from build123d import *

# Parameters (mm, degrees)
CYLINDER072_R               = 42
CYLINDER072_DEPTH           = 297
CYLINDER073_W               = 46
CYLINDER073_H               = 280
CYLINDER073_ANGLE           = 230
CYLINDER073_PLACEMENT_ANGLE = 184


with BuildPart() as cylindre068:
    # Cylinder072 → Cylinder072 (new body)
    with BuildSketch(Plane.XY.offset(-207)):
        Circle(CYLINDER072_R)
    extrude(amount=CYLINDER072_DEPTH)


with BuildPart() as obj1:
    # Cylinder073 → Cylinder073 (revolve)
    with BuildSketch(Plane.XZ):
        with Locations((23, 140)):
            Rectangle(CYLINDER073_W, CYLINDER073_H)
    revolve(axis=Axis((0, 0, 0), (0, 0, 1)), revolution_arc=CYLINDER073_ANGLE)


with BuildPart() as obj1_1:
    # Cylinder073 placement: moved
    add(obj1.part.moved(Location((0, 0, -207))).rotate(Axis((0, 0, -207), (0, 0, 1)), CYLINDER073_PLACEMENT_ANGLE))

    # Cut041: cut Cylindre068
    add(cylindre068.part, mode=Mode.SUBTRACT)


with BuildPart() as obj1_2:
    # Cut041 placement: moved
    add(obj1_1.part.moved(Location((0, 0, 8))))


solid = obj1_2.part
Can you work these out from the model? Positions are in its coordinate system, mm. Coordinates: 2 decimals unless noted, no trailing zeros. Loops run counter-clockwise (first coordinate to the right, second up) from the corner with the lowest first, then second, coordinate; pieces in that order, holes last. Notation, with made-up numbers: (62.25, -40) - (94.25, -40) arc R25 ccw to (94.25, -16) - close; hole circle Ø9 at (38.5, 15). An arc over 180 degrees is marked (long way). Put each result on its own line as item: value. Start each with the question number.
Item 1: If I drill on line 1 along Y through (x, z) = (0, -15.5); line 2 along X through (y, z) = (1, -125); line 3 along X through (y, z) = (-38.5, -93), over which ranges is the centre line in solid material (lowest first)?
Item 2: Suppose I cut it at A-A (y = -11.5). Please give me the cut outline in (x, z), and give its area (3 significant figures).
Item 3: If we mould it in two halves opening along X, with no side actions, what happens to faces 1 (the face through (19.5, -37.4, 81)), 2 (the face through (21.162, -40.843, -57.04)), 3 (the face through (19.322, -37.292, -60.96))? For each: +X half, -X half, draft (parallel to the pull), parting line (faces both ways), or undercut.
Item 4: For pin 1 (3 mm diameter, centred on y = -11.5, z = -24, fed in from -X); pin 2 (6 mm diameter, centred on y = 23, z = -4.5, fed in from +X); pin 3 (12 mm diameter, centred on x = -16, z = -158.5, fed in from -Y), each with a flat end and sliding along its axis, tell me the tip position at first contact or that it passes through.
Item 5: Suppose I cut it at C-C (x = 0). Please give me the cut outline in (y, z), and give its area (3 significant figures).
Item 6: Suppose I cut it at D-D (z = -137). Please give me the cut outline in (x, y).
Item 7: Suppose I cut it at B-B (x = 39.5). Please give me the cut outline in (y, z), and give its area (3 significant figures).
Here are the results:
1. line 1: -46 to -42
1. line 2: 41.99 to 45.99
1. line 3: -25.17 to -16.79, 16.79 to 25.17
2. outline: (-44.54, -199) - (-40.39, -199) - (-40.39, 81) - (-44.54, 81) - close; (40.39, -199) - (44.54, -199) - (44.54, 81) - (40.39, 81) - close
2. area: 2,320 mm²
3. face 1: draft
3. face 2: parting line
3. face 3: undercut
4. pin 1: x = -44.9
4. pin 2: x = 41.42
4. pin 3: y = -44.9
5. outline: (-46, -199) - (-42, -199) - (-42, 81) - (-46, 81) - close
5. area: 1,120 mm²
6. outline: (-45.89, -3.21) arc R46 ccw (long way) to (27.04, 37.21) - (24.69, 33.98) arc R42 cw (long way) to (-41.9, -2.93) - close
7. outline: (-23.57, -199) - (-14.27, -199) - (-14.27, 81) - (-23.57, 81) - close; (14.27, -199) - (23.57, -199) - (23.57, 81) - (14.27, 81) - close
7. area: 5,210 mm²
